Source: CAD feature listing. Evaluate the final solid. Frame: model axes, mm. Give positions to 0.01 mm unless a question says otherwise; leave off trailing zeros. Write each loop counter-clockwise with the first axis right and the second up, starting at its lowest first coordinate (ties: lowest second). Pieces come first, ordered by that corner, then holes. Notation, with made-up numbers: (-36.5, 56.25) -> (-0.5, 56.25) arc R17 ccw to (-0.5, 60.25) -> close; hole circle Ø9 at (-24, 33.25). An arc over 180 degrees is marked (long way). Use a Markdown table: item, result. Add a question column.
```python
from build123d import *

# Parameters (mm, degrees)
SKETCH1_W               = 381
SKETCH1_H               = 152.4
BOSS_EXTRUDE1_DEPTH     = 6.35
SKETCH2_W               = 69.85
SKETCH2_H               = 6.35
CUT_EXTRUDE2_DEPTH      = 7.35
LPATTERN1_COUNT         = 3
LPATTERN1_PITCH         = 95.25
LPATTERN1_COL_COUNT     = 3
LPATTERN1_COL_PITCH     = 95.25
MIRROR2_COPY_1_SKETCH_W = 69.85
MIRROR2_COPY_1_SKETCH_H = 6.35
MIRROR2_COPY_1_DEPTH    = 7.35
MIRROR2_COPY_2_SKETCH_W = 69.85
MIRROR2_COPY_2_SKETCH_H = 6.35
MIRROR2_COPY_2_DEPTH    = 7.35
MIRROR2_COPY_3_SKETCH_W = 69.85
MIRROR2_COPY_3_SKETCH_H = 6.35
MIRROR2_COPY_3_DEPTH    = 7.35
MIRROR2_COPY_4_SKETCH_W = 69.85
MIRROR2_COPY_4_SKETCH_H = 6.35
MIRROR2_COPY_4_DEPTH    = 7.35


with BuildPart() as part:
    # Sketch1 → Boss-Extrude1 (new body)
    with BuildSketch(Plane(origin=(0, 0, 0), x_dir=(1, 0, 0), z_dir=(0, 1, 0))):
        Rectangle(SKETCH1_W, SKETCH1_H)
    extrude(amount=BOSS_EXTRUDE1_DEPTH)

    # Sketch2 → Cut-Extrude2 (cut, through all)
    with BuildSketch(Plane(origin=(0, 6.35, 0), x_dir=(1, 0, 0), z_dir=(0, 1, 0))):
        with Locations((0, -73.025)):
            Rectangle(SKETCH2_W, SKETCH2_H)
    cut_extrude2 = extrude(amount=-CUT_EXTRUDE2_DEPTH, mode=Mode.SUBTRACT)

    # LPattern1: Cut-Extrude2 ×3
    with Locations(*[(-i * LPATTERN1_PITCH, 0, 0) for i in range(1, LPATTERN1_COUNT)]):
        add(cut_extrude2, mode=Mode.SUBTRACT)

    # LPattern1 col: Cut-Extrude2 ×3
    with Locations(*[(i * LPATTERN1_COL_PITCH, 0, 0) for i in range(1, LPATTERN1_COL_COUNT)]):
        add(cut_extrude2, mode=Mode.SUBTRACT)

    # Mirror2: Cut-Extrude2 across plane
    add(cut_extrude2.mirror(Plane.XY), mode=Mode.SUBTRACT)

    # Mirror2 copy 1 sketch → Mirror2 copy 1 (cut, through all)
    with BuildSketch(Plane(origin=(-95.25, 6.35, 0), x_dir=(1, 0, 0), z_dir=(0, 1, 0))):
        with Locations((0, 73.025)):
            Rectangle(MIRROR2_COPY_1_SKETCH_W, MIRROR2_COPY_1_SKETCH_H)
    extrude(amount=-MIRROR2_COPY_1_DEPTH, mode=Mode.SUBTRACT)

    # Mirror2 copy 2 sketch → Mirror2 copy 2 (cut, through all)
    with BuildSketch(Plane(origin=(-190.5, 6.35, 0), x_dir=(1, 0, 0), z_dir=(0, 1, 0))):
        with Locations((0, 73.025)):
            Rectangle(MIRROR2_COPY_2_SKETCH_W, MIRROR2_COPY_2_SKETCH_H)
    extrude(amount=-MIRROR2_COPY_2_DEPTH, mode=Mode.SUBTRACT)

    # Mirror2 copy 3 sketch → Mirror2 copy 3 (cut, through all)
    with BuildSketch(Plane(origin=(95.25, 6.35, 0), x_dir=(1, 0, 0), z_dir=(0, 1, 0))):
        with Locations((0, 73.025)):
            Rectangle(MIRROR2_COPY_3_SKETCH_W, MIRROR2_COPY_3_SKETCH_H)
    extrude(amount=-MIRROR2_COPY_3_DEPTH, mode=Mode.SUBTRACT)

    # Mirror2 copy 4 sketch → Mirror2 copy 4 (cut, through all)
    with BuildSketch(Plane(origin=(190.5, 6.35, 0), x_dir=(1, 0, 0), z_dir=(0, 1, 0))):
        with Locations((0, 73.025)):
            Rectangle(MIRROR2_COPY_4_SKETCH_W, MIRROR2_COPY_4_SKETCH_H)
    extrude(amount=-MIRROR2_COPY_4_DEPTH, mode=Mode.SUBTRACT)


solid = part.part
```
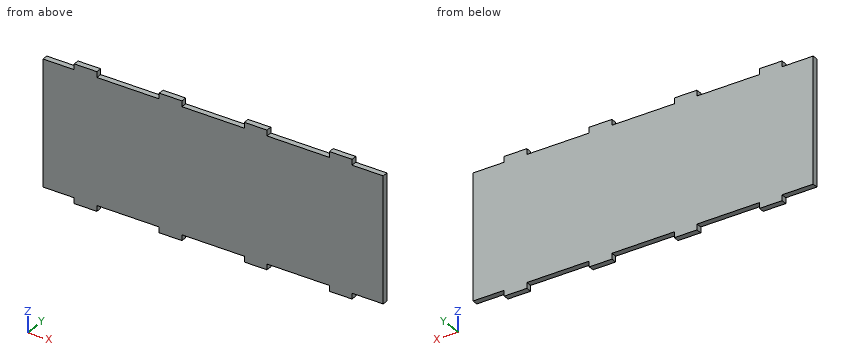
(1) First-contact query: pin 1 Ø1 at (x, y) = (-74.5, 2.5) entering from -Z; pin 2 Ø3 at (y, z) = (4.5, 73.5) entering from -X (3 decimals); pin 3 Ø1.9 at (y, z) = (3, -74) entering from +X (3 decimals). Flat tips, straight axial feed; report the tip coordinate or a pass-through.
(2) Material intervals for L1, parallel to Z at x = -15, y = 5.25, sorted ascending.
(3) Cut plane A-A on x = 72.5. Return the cut outline in (y, z), then the cut area to 3 significant figures.
Output:
| question | item | result |
|---|---|---|
| 1 | pin 1 | z = -69.85 |
| 1 | pin 2 | x = -155.575 |
| 1 | pin 3 | x = 155.575 |
| 2 | L1 | -69.85 to 69.85 |
| 3 | outline | (0, -69.85) -> (6.35, -69.85) -> (6.35, 69.85) -> (0, 69.85) -> close |
| 3 | area | 887 mm^2 |
